Autodesk Inventor part; units mm, degrees
ref_plane "YZ Plane" through (0, 0, 0) normal (1, 0, 0) x (0, 1, 0)
ref_plane "XZ Plane" through (0, 0, 0) normal (0, 1, 0) x (-1, 0, 0)
ref_plane "XY Plane" through (0, 0, 0) normal (0, 0, 1) x (1, 0, 0)
sketch "Szkic1" plane through (0, 0, 0) normal (0, 1, 0) x (-1, 0, 0)
  circle A0 centre (0, 0) radius 13.5
  dimension "d0" = 27
extrude "Wyciągnięcie proste1" add sketch "Szkic1" along normal blind 1
sketch "Szkic2" plane through (0, 1, 0) normal (0, 1, 0) x (1, 0, 0)
  circle A0 centre (0, 0) radius 12.5
  dimension "d3" = 25
extrude "Wyciągnięcie proste2" add sketch "Szkic2" along normal blind 5.5
sketch "Szkic3" plane through (0, 6.5, 0) normal (0, 1, 0) x (1, 0, 0)
  point P0 (0, 0)
  point P1 (1.5, -6.75)
  point P2 (1.5, 6.75)
  dimension "d21" = 6.75
hole "Otwór1" at (1.5, 6.5, 6.75) at (1.5, 6.5, -6.75) direction (0, -1, 0) diameter 3.2 end through all
sketch "Szkic5" plane through (0, 0, 0) normal (0, -1, 0) x (1, 0, 0)
  arc A0 (-0.62, -1.59) -> (-0.62, 1.59) centre (1.5, 0) ccw
  line L0 (-0.62, 1.59) -> (-0.62, -1.59)
  point P0 (0, 0)
  dimension "d16" = 5.3
extrude "Wyciągnięcie proste3" cut sketch "Szkic5" against normal through all
properties part number "RotorShaft2"
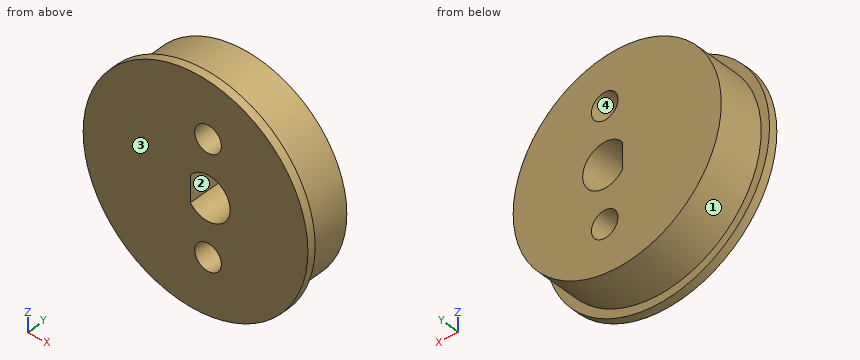
Could you check a few things on this model? Use its own coordinates, in mm. Face numbers are marked on the shaded views. Round coordinates to 2 decimals unless told otherwise and drop trailing zeros. Loops run counter-clockwise (first coordinate to the right, second up) from the corner with the lowest first, then second, coordinate; pieces in that order, holes last. Notation, with made-up numbers: (69, 83) - (78, 83) arc R26 ccw to (78, 109) - close; hole circle Ø1 at (47, -32). An arc over 180 degrees is marked (long way). Answer in a Markdown table with one row per item. Add a question column.
(1) If we section it at B-B (z = 0): Please give me the cut outline in (x, y).
(2) If we section it at C-C (y = 4.25): Please give me the cut outline in (x, z).
(3) I need wall thicknesses on line 1 along X through (y, z) = (4.75, 0); line 2 along Z through (x, y) = (1.5, 4.75); line 3 along Y through (x, z) = (-4.25, 12.25). Which ranges of each line are inside material? Lowest first, please.
(4) If we section it at A-A (x = 1.5): Please give me the cut outline in (y, z), plus the area to 3 significant figures.
(5) If we section it at D-D (z = 12): Please give me the cut outline in (x, y).
(6) If we mould it in two halves opening along X, with no side actions, what happens to the marked faces 1, 2, 3 and 4? For each: pulls with the +X half, pulls with the -X half, needs draft (parallel to the pull), parting line crosses it, or undercut.
(7) I'm going to push flat-ended pins straight in: pin 1 (1.5 mm diameter, centred on x = 1.5, y = 2, fed in from +Z); pin 2 (1 mm diameter, centred on y = 3.5, z = -0.5, fed in from +X); pin 3 (1.5 mm diameter, centred on y = 4, z = -8.5, fed in from -X). Where does each tip first touch, or does it pass through?
Model answer:
| question | item | result |
|---|---|---|
| 1 | outline | (-13.5, 0) - (-0.62, 0) - (-0.62, 6.5) - (-12.5, 6.5) - (-12.5, 1) - (-13.5, 1) - close; (4.15, 0) - (13.5, 0) - (13.5, 1) - (12.5, 1) - (12.5, 6.5) - (4.15, 6.5) - close |
| 2 | outline | circle Ø25 at (0, 0); hole (-0.62, -1.59) arc R2.65 ccw (long way) to (-0.62, 1.59) - close; hole circle Ø3.2 at (1.5, -6.75); hole circle Ø3.2 at (1.5, 6.75) |
| 3 | line 1 | x = -12.5 to -0.62, 4.15 to 12.5 |
| 3 | line 2 | z = -12.41 to -8.35, -5.15 to -2.65, 2.65 to 5.15, 8.35 to 12.41 |
| 3 | line 3 | y = 0 to 1 |
| 4 | outline | (0, -13.42) - (1, -13.42) - (1, -12.41) - (6.5, -12.41) - (6.5, -8.35) - (0, -8.35) - close; (0, -5.15) - (6.5, -5.15) - (6.5, -2.65) - (0, -2.65) - close; (0, 2.65) - (6.5, 2.65) - (6.5, 5.15) - (0, 5.15) - close; (0, 8.35) - (6.5, 8.35) - (6.5, 12.41) - (1, 12.41) - (1, 13.42) - (0, 13.42) - close |
| 4 | area | 87.3 mm² |
| 5 | outline | (-6.18, 0) - (6.18, 0) - (6.18, 1) - (3.5, 1) - (3.5, 6.5) - (-3.5, 6.5) - (-3.5, 1) - (-6.18, 1) - close |
| 6 | face 1 | parting line crosses it |
| 6 | face 2 | undercut |
| 6 | face 3 | needs draft |
| 6 | face 4 | undercut |
| 7 | pin 1 | stops at z = 12.48 |
| 7 | pin 2 | stops at x = 12.5 |
| 7 | pin 3 | stops at x = -9.81 |
